from build123d import *

# Parameters (mm, degrees)
SKETCH1_R           = 22.86
BOSS_EXTRUDE1_DEPTH = 22.86
SKETCH3_R           = 15.24
BOSS_EXTRUDE2_DEPTH = 55.88
SKETCH4_R           = 22.86
BOSS_EXTRUDE3_DEPTH = 22.86
FILLET3_R           = 2.54
CUT_EXTRUDE1_DEPTH  = 102.6
FILLET4_R           = 1


with BuildPart() as part:
    # Sketch1 → Boss-Extrude1 (new body)
    with BuildSketch(Plane(origin=(0, 0, 0), x_dir=(1, 0, 0), z_dir=(0, 1, 0))):
        Circle(SKETCH1_R)
    extrude(amount=BOSS_EXTRUDE1_DEPTH)

    # Sketch3 → Boss-Extrude2 (add)
    with BuildSketch(Plane(origin=(0, 22.86, 0), x_dir=(1, 0, 0), z_dir=(0, 1, 0))):
        Circle(SKETCH3_R)
    extrude(amount=BOSS_EXTRUDE2_DEPTH)

    # Sketch4 → Boss-Extrude3 (add)
    with BuildSketch(Plane(origin=(0, 78.74, 0), x_dir=(1, 0, 0), z_dir=(0, 1, 0))):
        Circle(SKETCH4_R)
    extrude(amount=BOSS_EXTRUDE3_DEPTH)

    # Fillet3
    fillet3_edges = [part.edges().sort_by_distance(p)[0] for p in [
        (-22.86, 101.6, 0),
        (-22.86, 0, 0),
    ]]
    fillet(fillet3_edges, radius=FILLET3_R)

    # Sketch5 → Cut-Extrude1 (cut, through all)
    with BuildSketch(Plane(origin=(0, 101.6, 0), x_dir=(1, 0, 0), z_dir=(0, 1, 0))):
        Polygon((-1.8, -0.03), (-1.8, -1.7), (1.8, -1.7), (1.8, 1.64), (-1.8, 1.64), align=None)
    extrude(amount=-CUT_EXTRUDE1_DEPTH, mode=Mode.SUBTRACT)

    # Fillet4
    fillet4_edges = [part.edges().sort_by_distance(p)[0] for p in [
        (0, 0, -1.64),
        (1.8, 0, 0.03),
        (0, 0, 1.7),
        (-1.8, 0, 0.03),
        (0, 101.6, -1.64),
        (-1.8, 101.6, 0.03),
        (0, 101.6, 1.7),
        (1.8, 101.6, 0.03),
    ]]
    fillet(fillet4_edges, radius=FILLET4_R)


solid = part.part
Design review of the part built by this model. Coordinates are the model's own, in mm. A direction names the side the tool comes from. Round coordinates to 2 decimals unless told otherwise and drop trailing zeros. Loops run counter-clockwise (first coordinate to the right, second up) from the corner with the lowest first, then second, coordinate; pieces in that order, holes last. Notation, with made-up numbers: M 51.5,-31.75 L 55.5,-31.75 A19 cw 55.5,-17.75 Z; hole C 46.5,20 d6. An arc over 180 degrees is marked long. Answer as a JSON object with one key per item and string values.
Item 1: We need section B-B on z = 0. Give the boundary of the cut face in (x, y), and give its area (3 significant figures).
Answer sheet:
{"outline": "M -22.86,2.54 A2.54 ccw -20.32,0 L -2.8,0 A1 ccw -1.8,1 L -1.8,100.6 A1 ccw -2.8,101.6 L -20.32,101.6 A2.54 ccw -22.86,99.06 L -22.86,78.74 L -15.24,78.74 L -15.24,22.86 L -22.86,22.86 Z; M 1.8,1 A1 ccw 2.8,0 L 20.32,0 A2.54 ccw 22.86,2.54 L 22.86,22.86 L 15.24,22.86 L 15.24,78.74 L 22.86,78.74 L 22.86,99.06 A2.54 ccw 20.32,101.6 L 2.8,101.6 A1 ccw 1.8,100.6 Z", "area": "3,420 mm^2"}
Item 2: Machinability: for faces 1 (the flat face through (5, 22.86, 15)), 2 (the flat face through (0, 51, -1.64)), 3 (the flat face through (0, 101.6, 4)), which of the approach directions +Z, -Z, +X, -X, +Y, -Y give a long, thin tool a straight path to every point of the face, cutting with its end or side? Answer none if there is none.
Answer sheet:
{"face 1": "none", "face 2": "+Y, -Y", "face 3": "+Z, -Z, +X, -X, +Y"}
Item 3: Clearance check with flat-ended pins moving along their axes: P1, Ø1, axis at y = 35, z = -0.5, coming from the +X side; P2, Ø6, axis at y = 32.5, z = -3.5, coming from the -X side; P3, Ø4, axis at x = 0, y = 40, coming from the -Z side. State where each tip first meets the part, or that it passes through.
Answer sheet:
{"P1": "stops at x = 15.24", "P2": "stops at x = -15.23", "P3": "stops at z = -15.24"}
Item 4: Wall thickness on L1, parallel to Y at x = 17.5, z = -4; L2, parallel to Y at x = 17, z = -14.5; L3, parallel to Z at x = -0.5, y = 70.5: over which ranges is each line inside the solid? List them lowest first. Write a range as from..to.
Answer sheet:
{"L1": "y = 0..22.86, 78.74..101.6", "L2": "y = 1.01..22.86, 78.74..100.59", "L3": "z = -15.23..-1.64, 1.7..15.23"}
Item 5: We need section A-A on x = 0. Give the boundary of the cut face in (y, z).
Answer sheet:
{"outline": "M 0,-20.32 A2.54 ccw 2.54,-22.86 L 22.86,-22.86 L 22.86,-15.24 L 78.74,-15.24 L 78.74,-22.86 L 99.06,-22.86 A2.54 ccw 101.6,-20.32 L 101.6,-2.64 A1 ccw 100.6,-1.64 L 1,-1.64 A1 ccw 0,-2.64 Z; M 0,2.7 A1 ccw 1,1.7 L 100.6,1.7 A1 ccw 101.6,2.7 L 101.6,20.32 A2.54 ccw 99.06,22.86 L 78.74,22.86 L 78.74,15.24 L 22.86,15.24 L 22.86,22.86 L 2.54,22.86 A2.54 ccw 0,20.32 Z"}
Item 6: We need section D-D on y = 65.5. Give the boundary of the cut face in (x, z), and give its area (3 significant figures).
Answer sheet:
{"outline": "C 0,0 d30.48; hole M -1.8,-1.64 L 1.8,-1.64 L 1.8,1.7 L -1.8,1.7 Z", "area": "718 mm^2"}
Item 7: We need section C-C on y = 18. Give the boundary of the cut face in (x, z).
Answer sheet:
{"outline": "C 0,0 d45.72; hole M -1.8,-1.64 L 1.8,-1.64 L 1.8,1.7 L -1.8,1.7 Z"}
Item 8: The part is to be moulded in two halves that separate along X. For faces 4 (the flat face through (0, 0, 4)), 5 (the cylindrical face through (-3.3, 50.41, 14.88)), 6 (the flat face through (-1.8, 51, 0)), say which applies: pulls with the +X half, pulls with the -X half, needs draft (parallel to the pull), parting line crosses it, or undercut.
Answer sheet:
{"face 4": "needs draft", "face 5": "parting line crosses it", "face 6": "undercut"}
